Input: part model. Units: mm. Frame: model coordinates. Face numbers are marked on the shaded views. A direction names the side the tool comes from. Round coordinates to 2 decimals unless told otherwise and drop trailing zeros. Order: outer loops, then holes, each group sorted by start corner. A loop starts at its lowest first (then second) coordinate and runs counter-clockwise, first axis right, second up. Notation, with made-up numbers: M 29.5,-28 L 55.5,-28 A33 ccw 55.5,4 Z; hole C 16.5,63.25 d3. An arc over 180 degrees is marked long. One line per question, with ' | ' between items.
```python
from build123d import *

# Parameters (mm, degrees)
BOX013_W            = 1
BOX013_H            = 3.2
BOX013_DEPTH        = 3
CYLINDER009_R       = 4.15
CYLINDER009_DEPTH   = 10
CYLINDER007_R       = 4.15
CYLINDER007_DEPTH   = 10
BOX007_W            = 50
BOX007_H            = 25
BOX007_DEPTH        = 0.5
SKETCH006_R         = 15
EXTRUDE003003_DEPTH = 17.25


with BuildPart() as cube012:
    # Box013 → Box013 (new body)
    with BuildSketch(Plane(origin=(88.5, -17.3, 9), x_dir=(1, 0, 0), z_dir=(0, 0, 1))):
        with Locations((0.5, 1.6)):
            Rectangle(BOX013_W, BOX013_H)
    extrude(amount=BOX013_DEPTH)


with BuildPart() as obj1:
    # Cylinder009 → Cylinder009 (new body)
    with BuildSketch(Plane(origin=(93.2, -14.9, 10.4), x_dir=(1, 0, 0), z_dir=(0, -1, 0))):
        Circle(CYLINDER009_R)
    extrude(amount=CYLINDER009_DEPTH)


with BuildPart() as obj2:
    # Cylinder007 → Cylinder007 (new body)
    with BuildSketch(Plane(origin=(84.8, -13.9, 10.4), x_dir=(1, 0, 0), z_dir=(0, -1, 0))):
        Circle(CYLINDER007_R)
    extrude(amount=CYLINDER007_DEPTH)


with BuildPart() as cube007:
    # Box007 → Box007 (new body)
    with BuildSketch(Plane(origin=(66, 0, -2), x_dir=(1, 0, 0), z_dir=(0, -1, 0))):
        with Locations((25, 12.5)):
            Rectangle(BOX007_W, BOX007_H)
    extrude(amount=BOX007_DEPTH)


with BuildPart() as obj3:
    # Sketch006 → Extrude003003 (new body)
    with BuildSketch(Plane.XZ):
        with Locations((89, 10.4)):
            Circle(SKETCH006_R)
    extrude(amount=EXTRUDE003003_DEPTH)

    # Cut005014006: cut Cube007
    add(cube007.part, mode=Mode.SUBTRACT)

    # Cut005014007: cut obj2
    add(obj2.part, mode=Mode.SUBTRACT)

    # Cut005014010: cut obj1
    add(obj1.part, mode=Mode.SUBTRACT)

    # Cut005014011: cut Cube012
    add(cube012.part, mode=Mode.SUBTRACT)


solid = obj3.part
```
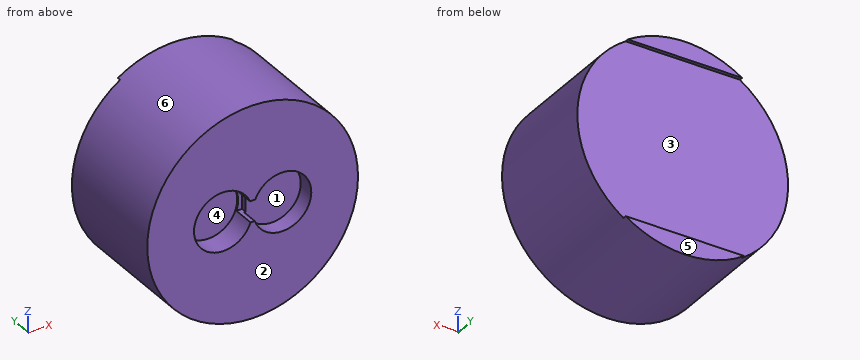
Item 1: Line query: line 1 along X through (y, z) = (-15.8, 10.4); line 2 along Y through (x, z) = (95.5, 14.25); line 3 along Z through (x, y) = (93.2, -16.35). Output: solid intervals per line, ascending. Write a range as from..to.
Report:
line 1: 74..80.65, 97.35..104 | line 2: -17.25..-0.5 | line 3: -4..6.25, 14.55..24.8
Item 2: Section query A-A, the plane x = 84.8. Return loops of the section in (y, z).
Report:
outline: M -17.25,-4 L 0,-4 L 0,-2 L -0.5,-2 L -0.5,23 L 0,23 L 0,24.8 L -17.25,24.8 L -17.25,14.55 L -13.9,14.55 L -13.9,6.25 L -17.25,6.25 Z
Item 3: Access query for the marked faces 1, 2 and 3. Directions: +Z, -Z, +X, -X, +Y, -Y. A direction counts if a zero-diameter tool reaches every point of the face in a straight line with its end or side. Return the directions, or none.
Report:
face 1: -Y | face 2: +Z, -Z, +X, -X, -Y | face 3: +X, -X, +Y
Item 4: Section query B-B, the plane z = 10.4. Return loops of the section in (x, y).
Report:
outline: M 74,-17.25 L 80.65,-17.25 L 80.65,-13.9 L 88.95,-13.9 L 88.95,-14.1 L 89.5,-14.1 L 89.5,-14.9 L 97.35,-14.9 L 97.35,-17.25 L 104,-17.25 L 104,-0.5 L 74,-0.5 Z
Item 5: Section query C-C, the plane y = -10.75. Return loops of the section in (x, z).
Report:
outline: C 89,10.4 d30
Item 6: First-contact query: pin 1 (1.5 mm diameter, centred on y = -4.5, z = -1, fed in from +X); pin 2 (4 mm diameter, centred on x = 97.5, y = -11.5, fed in from +Z); pin 3 (0.6 mm diameter, centred on x = 92.5, y = 0, fed in from -Z); pin 4 (5 mm diameter, centred on x = 89.5, z = 9.5, fed in from -Y). Flat tips, straight axial feed; report the tip coordinate or a pass-through.
Report:
pin 1: x = 99.56 | pin 2: z = 23.92 | pin 3: z = -4.25 | pin 4: y = -17.25
Item 7: Section query D-D, the plane z = 22. Return loops of the section in (x, y), plus the area to 3 significant figures.
Report:
outline: M 79.49,-17.25 L 98.51,-17.25 L 98.51,-0.5 L 79.49,-0.5 Z | area: 319 mm²
Item 8: Mould query, pull axis Z, two halves, no side actions, for the marked faces 4, 5 and 6. Classes: +Z half, -Z half, draft (parallel to the pull), parting line (faces both ways), or undercut.
Report:
face 4: undercut | face 5: draft | face 6: parting line
